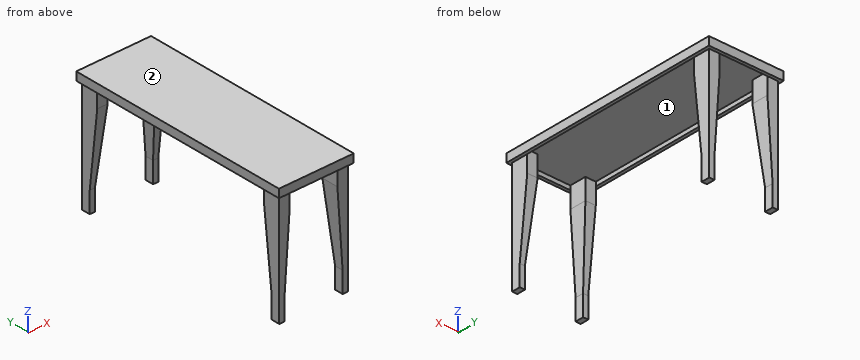
from build123d import *

# Parameters (mm, degrees)
F0_W     = 457.2
F0_H     = 1371.6
F0_W_2   = 419.1
F0_H_2   = 1333.5
F1_DEPTH = 25.4
F2_W     = 457.2
F2_H     = 1371.6
F3_DEPTH = 25.4
F4_W     = 63.5
F4_H     = 101.6
F5_DEPTH = 711.2
F7_DEPTH = 1352.551
F9_DEPTH = 438.151


with BuildPart() as f1:
    # F0 (on Top) → F1 (new body)
    with BuildSketch(Plane.XY):
        with Locations((228.6, 685.8)):
            Rectangle(F0_W, F0_H)
        with Locations((228.6, 685.8)):
            Rectangle(F0_W_2, F0_H_2, mode=Mode.SUBTRACT)
    extrude(amount=F1_DEPTH)

    # F2 (on face) → F3 (join)
    with BuildSketch(Plane.XY.offset(25.4)):
        with Locations((228.6, 685.8)):
            Rectangle(F2_W, F2_H)
    extrude(amount=F3_DEPTH)

    # F4 (on face) → F5 (join)
    with BuildSketch(Plane(origin=(0, 0, 25.4), x_dir=(1, 0, 0), z_dir=(0, 0, -1))):
        with Locations((50.8, -69.85)):
            Rectangle(F4_W, F4_H)
        with Locations((406.4, -69.85)):
            Rectangle(F4_W, F4_H)
        with Locations((50.8, -1301.75)):
            Rectangle(F4_W, F4_H)
        with Locations((406.4, -1301.75)):
            Rectangle(F4_W, F4_H)
    extrude(amount=F5_DEPTH)

    # F6 (on face) → F7 (cut, through all)
    with BuildSketch(Plane.XZ.offset(-19.05)):
        Polygon((50.8, -558.8), (50.8, -685.8), (406.4, -685.8), (406.4, -558.8), (374.65, -101.6), (82.55, -101.6), align=None)
    extrude(amount=-F7_DEPTH, mode=Mode.SUBTRACT)

    # F8 (on face) → F9 (cut, through all)
    with BuildSketch(Plane.YZ.offset(438.15)):
        Polygon((69.85, -558.8), (69.85, -685.8), (1301.75, -685.8), (1301.75, -558.8), (1250.95, -101.6), (120.65, -101.6), align=None)
    extrude(amount=-F9_DEPTH, mode=Mode.SUBTRACT)


solid = f1.part
Read the model definition and answer for the solid it produces. Units are mm, in the model's axes. Face numbers are marked on the shaded views. Give positions to 0.01 mm unless a question says otherwise; leave off trailing zeros. Write each loop counter-clockwise with the first axis right and the second up, starting at its lowest first coordinate (ties: lowest second). Pieces come first, ordered by that corner, then holes. Notation, with made-up numbers: (-16, -4.75) - (27, -4.75) arc R28 ccw to (27, 34.25) - close; hole circle Ø8 at (52, -17). An arc over 180 degrees is marked (long way). Use CSV: the item, a comma, the result in double quotes. Start each with the question number.
(1) Find section D-D (z = -371). Give the vertices of the cut face in (x, y), plus the area to 3 significant figures.
(2) Determine the mould class of the marked faces 1 and 2 for opening direction X: +X half, -X half, draft (parallel to the pull), parting line (faces both ways), or undercut.
(3) Given P1, Ø1, axis at x = 100.5, y = 974.5, coming from the -Z side; P2, Ø12, axis at x = 72.5, z = -41, coming from the +Y side; P3, Ø9.5, axis at x = 417.5, z = -612, coming from the -Y side, each flat-ended and moving along its own axis, determine where each tip first touches the part or whether it passes through.
(4) Find section A-A (z = -630.5). Give the vertices of the cut face in (x, y).
(5) Find section B-B (x = 179.5). Give the vertices of the cut face in (y, z).
(6) Find section C-C (y = 976). Give the vertices of the cut face in (x, z).
(7) Consider line 1 along Z through (x, y) = (312.5, 1088.5); line 2 along X through (y, z) = (1311, -110); line 3 along Y through (x, z) = (411, -105). Determine where each line is inside the solid, lowest interval first.
Findings below:
1,outline,"(19.05, 19.05) - (63.84, 19.05) - (63.84, 90.72) - (19.05, 90.72) - close; (19.05, 1280.88) - (63.84, 1280.88) - (63.84, 1352.55) - (19.05, 1352.55) - close; (393.36, 19.05) - (438.15, 19.05) - (438.15, 90.72) - (393.36, 90.72) - close; (393.36, 1280.88) - (438.15, 1280.88) - (438.15, 1352.55) - (393.36, 1352.55) - close"
1,area,"12,800 mm2"
2,face 1,"undercut"
2,face 2,"draft"
3,P1,"z = 25.4"
3,P2,"y = 1352.55"
3,P3,"y = 19.05"
4,outline,"(19.05, 19.05) - (50.8, 19.05) - (50.8, 69.85) - (19.05, 69.85) - close; (19.05, 1301.75) - (50.8, 1301.75) - (50.8, 1352.55) - (19.05, 1352.55) - close; (406.4, 19.05) - (438.15, 19.05) - (438.15, 69.85) - (406.4, 69.85) - close; (406.4, 1301.75) - (438.15, 1301.75) - (438.15, 1352.55) - (406.4, 1352.55) - close"
5,outline,"(0, 0) - (19.05, 0) - (19.05, 25.4) - (1352.55, 25.4) - (1352.55, 0) - (1371.6, 0) - (1371.6, 50.8) - (0, 50.8) - close"
6,outline,"(0, 0) - (19.05, 0) - (19.05, 25.4) - (438.15, 25.4) - (438.15, 0) - (457.2, 0) - (457.2, 50.8) - (0, 50.8) - close"
7,line 1,"25.4 to 50.8"
7,line 2,"19.05 to 81.97, 375.23 to 438.15"
7,line 3,"19.05 to 120.27, 1251.33 to 1352.55"
